Here's how the part is built. I have some questions about the finished solid (model axes, mm). Coordinates: 2 decimals unless noted, no trailing zeros. Loops run counter-clockwise (first coordinate to the right, second up) from the corner with the lowest first, then second, coordinate; pieces in that order, holes last. Notation, with made-up numbers: (87.5, 55.5) - (98.5, 55.5) arc R16 cw to (98.5, 78.5) - close; hole circle Ø4 at (-10.5, -37). An arc over 180 degrees is marked (long way). Use a Markdown table: item, result.
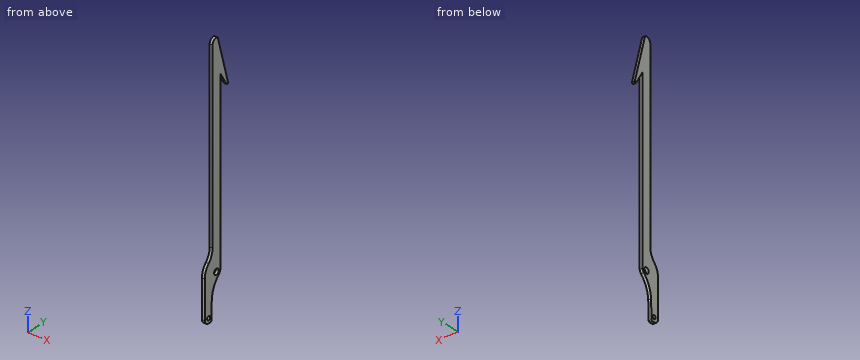
```python
from build123d import *

# Parameters (mm, degrees)
EXTRUDE_1_DEPTH     = 1.5
EXTRUDE_2_DEPTH     = 3
CUT_EXTRUDE_1_DEPTH = 226.519400496
SKETCH_4_W          = 70
SKETCH_4_H          = 10
EXTRUDE_3_DEPTH     = 3
CUT_EXTRUDE_2_DEPTH = 226.519400496
FILLET_1_R          = 5
FILLET_START        = -1.5
FILLET_2_DEPTH      = 3
FILLET_3_R          = 1
CUT_EXTRUDE_3_DEPTH = 226.519400496
SKETCH_7_R          = 3
CUT_EXTRUDE_4_DEPTH = 226.519400496
SKETCH_8_R          = 2
CUT_EXTRUDE_5_DEPTH = 226.519400496


with BuildPart() as part:
    # ｽｹｯﾁ1 → ﾎﾞｽ - 押し出し1 (new, symmetric)
    with BuildSketch(Plane(origin=(0, 0, 0), x_dir=(0, 0, -1), z_dir=(1, 0, 0))):
        with BuildLine():
            Line((0, -5), (-220, -5))
            ThreePointArc((-220, -5), (-225, 0), (-220, 5))
            Line((-220, 5), (0, 5))
            ThreePointArc((0, 5), (5, 0), (0, -5))
        make_face()
    extrude(amount=EXTRUDE_1_DEPTH, both=True)

    # ｽｹｯﾁ2 → ﾎﾞｽ - 押し出し2 (add)
    with BuildSketch(Plane(origin=(1.5, 0, 0), x_dir=(0, 0, -1), z_dir=(1, 0, 0))):
        with BuildLine():
            Line((-223.51763809, 1.931851653), (-174.873811044, 14.965925826))
            ThreePointArc((-174.873811044, 14.965925826), (-173.691112467, 14.382683432), (-174.114991999, 13.133974596))
            Line((-174.114991999, 13.133974596), (-196.863703305, 0))
            Line((-196.863703305, 0), (-225, 0))
            ThreePointArc((-225, 0), (-224.586706681, 1.217522858), (-223.51763809, 1.931851653))
        make_face()
    extrude(amount=-EXTRUDE_2_DEPTH)

    # ｽｹｯﾁ3 → ｶｯﾄ - 押し出し1 (cut, through all)
    with BuildSketch(Plane(origin=(1.5, 0, 0), x_dir=(0, 0, -1), z_dir=(1, 0, 0))):
        with BuildLine():
            Line((-223.51763809, 1.931851653), (-212.067152572, 5))
            Line((-212.067152572, 5), (-220, 5))
            ThreePointArc((-220, 5), (-223.535533906, 3.535533906), (-225, 0))
            ThreePointArc((-225, 0), (-224.586706681, 1.217522858), (-223.51763809, 1.931851653))
        make_face()
    extrude(amount=-CUT_EXTRUDE_1_DEPTH, mode=Mode.SUBTRACT)

    # ｽｹｯﾁ4 → ﾎﾞｽ - 押し出し3 (add)
    with BuildSketch(Plane(origin=(1.5, 0, 0), x_dir=(0, 0, -1), z_dir=(1, 0, 0))):
        with Locations((10, -10)):
            Rectangle(SKETCH_4_W, SKETCH_4_H)
    extrude(amount=-EXTRUDE_3_DEPTH)

    # ｽｹｯﾁ5 → ｶｯﾄ - 押し出し2 (cut, through all)
    with BuildSketch(Plane(origin=(1.5, 0, 0), x_dir=(0, 0, -1), z_dir=(1, 0, 0))):
        with BuildLine():
            ThreePointArc((-0.222112537, -4.995064166), (22.385361516, -5.899367469), (45, -6.602057872))
            Line((45, -6.602057872), (45, -5))
            Line((45, -5), (0, -5))
            ThreePointArc((0, -5), (-0.111083686, -4.998765889), (-0.222112537, -4.995064166))
        make_face()
    extrude(amount=-CUT_EXTRUDE_2_DEPTH, mode=Mode.SUBTRACT)

    # ﾌｨﾚｯﾄ1
    fillet_1_edges = [part.edges().sort_by_distance(p)[0] for p in [
        (0, -15, -45),
    ]]
    fillet(fillet_1_edges, radius=FILLET_1_R)

    # ﾌｨﾚｯﾄ2: read off the stored shape, not the designer's step
    # ﾌｨﾚｯﾄ2 outline → ﾌｨﾚｯﾄ2 (add)
    with BuildSketch(Plane.YZ.offset(FILLET_START)):
        with BuildLine():
            ThreePointArc((-5.97098694, -24.423877243), (-3.3233227, -13.102392567), (3.430133723, -3.637881615))
            ThreePointArc((3.430133723, -3.637881615), (-2.082580259, -4.54564181), (-4.995064166, 0.222112537))
            ThreePointArc((-4.995064166, 0.222112537), (-5.512971584, -12.099696561), (-5.97098694, -24.423877243))
        make_face()
    extrude(amount=FILLET_2_DEPTH)

    # ﾌｨﾚｯﾄ3
    fillet_3_edges = [part.edges().sort_by_distance(p)[0] for p in [
        (0, -6.602057872, -45),
    ]]
    fillet(fillet_3_edges, radius=FILLET_3_R)

    # ｽｹｯﾁ6 → ｶｯﾄ - 押し出し3 (cut, through all)
    with BuildSketch(Plane(origin=(1.5, 0, 0), x_dir=(0, 0, -1), z_dir=(1, 0, 0))):
        with BuildLine():
            Line((0, -15), (-25, -15))
            Line((-25, -15), (-25, -5))
            ThreePointArc((-25, -5), (-18.268543991, -6.296359978), (-12.5, -10))
            ThreePointArc((-12.5, -10), (-6.731456009, -13.703640022), (0, -15))
        make_face()
    extrude(amount=-CUT_EXTRUDE_3_DEPTH, mode=Mode.SUBTRACT)

    # ｽｹｯﾁ7 → ｶｯﾄ - 押し出し4 (cut, through all)
    with BuildSketch(Plane(origin=(1.5, 0, 0), x_dir=(0, 0, -1), z_dir=(1, 0, 0))):
        Circle(SKETCH_7_R)
    extrude(amount=-CUT_EXTRUDE_4_DEPTH, mode=Mode.SUBTRACT)

    # ｽｹｯﾁ8 → ｶｯﾄ - 押し出し5 (cut, through all)
    with BuildSketch(Plane(origin=(1.5, 0, 0), x_dir=(0, 0, -1), z_dir=(1, 0, 0))):
        with Locations((40, -10)):
            Circle(SKETCH_8_R)
    extrude(amount=-CUT_EXTRUDE_5_DEPTH, mode=Mode.SUBTRACT)


solid = part.part
```
Q1. I want a section at A-A, the plane x = -0.05. Write out the boundary of the cut face in (y, z) (3 decimals).
Check values:
| item | result |
|---|---|
| outline | (-15, -40) arc R5 ccw to (-10, -45) - (-7.576, -45) arc R1 ccw to (-6.576, -44.027) arc R2537.5 cw to (-5.971, -24.424) arc R30 cw to (3.43, -3.638) arc R5 ccw to (5, 0) - (5, 188.203) - (13.134, 174.115) arc R1 ccw to (14.966, 174.874) - (1.932, 223.518) arc R2 ccw to (0, 225) arc R5 ccw to (-5, 220) - (-5, 25) arc R18.125 cw to (-10, 12.5) arc R18.125 ccw to (-15, 0) - close; hole circle Ø4 at (-10, -40); hole circle Ø6 at (0, 0) |
Q2. Please list where these lines run through material, in increasing order: L1, parallel to Y at x = 0.95, z = 0; L2, parallel to Y at x = -1.3, z = 98.5; L3, parallel to Y at x = 0.25, z = -40. Write a range as from..to.
Check values:
| item | result |
|---|---|
| L1 | -15..-3, 3..5 |
| L2 | -5..5 |
| L3 | -15..-12, -8..-6.46 |
Q3. Will these pins go through, and if not, where does the flat tip stop? P1, Ø0.9, axis at x = -0.5, z = 110.5, coming from the -Y side; P2, Ø1.5, axis at x = -1, y = -11.5, coming from the +Z side; P3, Ø3.5, axis at y = 0, z = 0, coming from the -X side (3 decimals); P4, Ø1, axis at x = 0.5, z = 14.5, coming from the -Y side.
Check values:
| item | result |
|---|---|
| P1 | y = -5 |
| P2 | z = 11.66 |
| P3 | through |
| P4 | y = -8.72 |
Q4. I want a section at B-B, the plane z = 36. Write out the boundary of the cut face in (x, y).
Check values:
| item | result |
|---|---|
| outline | (-1.5, -5) - (1.5, -5) - (1.5, 5) - (-1.5, 5) - close |
Q5. I want a section at C-C, the plane z = -15.5. Write out the boundary of the cut face in (x, y), then the cut area to 3 significant figures.
Check values:
| item | result |
|---|---|
| outline | (-1.5, -15) - (1.5, -15) - (1.5, -4.29) - (-1.5, -4.29) - close |
| area | 32.1 mm^2 |
